Geometry check sheet. Reference: the model listing, model coordinates, mm. A direction names the side the tool comes from. Round coordinates to 2 decimals unless told otherwise and drop trailing zeros. Return JSON: item names as keys, results as strings.
```python
from build123d import *
from build123d.topology import SkipClean

# Parameters (mm, degrees)
SKETCH1_R                    = 27.5
BOSS_EXTRUDE1_DEPTH          = 2
SKETCH2_R                    = 25
BOSS_EXTRUDE2_DEPTH          = 6.5
SKETCH3_R                    = 13
CUT_EXTRUDE1_DEPTH           = 5
SKETCH4_R                    = 11.5
CUT_EXTRUDE2_DEPTH           = 8.5
CHAMFER1_SIZE                = 1
SKETCH5_R                    = 1.55
CUT_EXTRUDE3_DEPTH           = 8.5
SKETCH6_R                    = 3
CUT_EXTRUDE4_DEPTH           = 6
CHAMFER2_SIZE                = 1
CIRPATTERN1_COUNT            = 6
CHAMFER2_OF_CIRPATTERN1_SIZE = 1
SKETCH7_R                    = 1.55
CUT_EXTRUDE5_DEPTH           = 8.5
SKETCH8_R                    = 2.15
CUT_EXTRUDE6_DEPTH           = 4.5
CIRPATTERN2_COUNT            = 6
SKETCH9_R                    = 2.5
SKETCH9_R_2                  = 1.55
BOSS_EXTRUDE3_DEPTH          = 2
CIRPATTERN3_COUNT            = 6


with BuildPart() as part:
    # Sketch1 → Boss-Extrude1 (new body)
    with BuildSketch(Plane(origin=(0, 0, 0), x_dir=(1, 0, 0), z_dir=(0, 1, 0))):
        with Locations(Location((0, 0, 0), (0, 0, 270))):
            Circle(SKETCH1_R)
    extrude(amount=BOSS_EXTRUDE1_DEPTH)

    # Sketch2 → Boss-Extrude2 (add)
    with BuildSketch(Plane(origin=(0, 2, 0), x_dir=(1, 0, 0), z_dir=(0, 1, 0))):
        with Locations(Location((0, 0, 0), (0, 0, 90))):
            Circle(SKETCH2_R)
    extrude(amount=BOSS_EXTRUDE2_DEPTH)

    # Sketch3 → Cut-Extrude1 (cut)
    with BuildSketch(Plane(origin=(0, 8.5, 0), x_dir=(1, 0, 0), z_dir=(0, 1, 0))):
        with Locations(Location((0, 0, 0), (0, 0, 270))):
            Circle(SKETCH3_R)
    extrude(amount=-CUT_EXTRUDE1_DEPTH, mode=Mode.SUBTRACT)

    # Sketch4 → Cut-Extrude2 (cut)
    with BuildSketch(Plane(origin=(0, 8.5, 0), x_dir=(1, 0, 0), z_dir=(0, 1, 0))):
        with Locations(Location((0, 0, 0), (0, 0, 270))):
            Circle(SKETCH4_R)
    extrude(amount=-CUT_EXTRUDE2_DEPTH, mode=Mode.SUBTRACT)

    # Chamfer1
    chamfer1_edges = [part.edges().sort_by_distance(p)[0] for p in [
        (0, 8.5, -13),
        (0, 0, -11.5),
        (0, 0, -27.5),
        (0, 8.5, 25),
    ]]
    chamfer(chamfer1_edges, length=CHAMFER1_SIZE)

    # Sketch5 → Cut-Extrude3 (cut)
    with BuildSketch(Plane.XZ):
        with Locations(Location((0, 21, 0), (0, 0, 270))):
            Circle(SKETCH5_R)
    cut_extrude3 = extrude(amount=-CUT_EXTRUDE3_DEPTH, mode=Mode.SUBTRACT)

    # Sketch6 → Cut-Extrude4 (cut)
    with BuildSketch(Plane.XZ):
        with Locations(Location((0, 21, 0), (0, 0, 270))):
            Circle(SKETCH6_R)
    cut_extrude4 = extrude(amount=-CUT_EXTRUDE4_DEPTH, mode=Mode.SUBTRACT)

    # Chamfer2
    chamfer2_edges = [part.edges().sort_by_distance(p)[0] for p in [
        (0, 0, 24),
    ]]
    chamfer(chamfer2_edges, length=CHAMFER2_SIZE)

    # CirPattern1: Cut-Extrude3, Cut-Extrude4 ×6 about axis
    cirpattern1_axis = Axis((0, 0, 0), (0, 1, 0))
    add([cut_extrude3.rotate(cirpattern1_axis, i * 360 / CIRPATTERN1_COUNT) for i in range(1, CIRPATTERN1_COUNT)], mode=Mode.SUBTRACT)
    add([cut_extrude4.rotate(cirpattern1_axis, i * 360 / CIRPATTERN1_COUNT) for i in range(1, CIRPATTERN1_COUNT)], mode=Mode.SUBTRACT)

    # Chamfer2 of CirPattern1
    chamfer2_of_cirpattern1_edges = [part.edges().sort_by_distance(p)[0] for p in [
        (20.784609691, 0, 12),
        (20.784609691, 0, -12),
        (0, 0, -24),
        (-20.784609691, 0, -12),
        (-20.784609691, 0, 12),
    ]]
    chamfer(chamfer2_of_cirpattern1_edges, length=CHAMFER2_OF_CIRPATTERN1_SIZE)

    # Sketch7 → Cut-Extrude5 (cut)
    with BuildSketch(Plane(origin=(0, 8.5, 0), x_dir=(1, 0, 0), z_dir=(0, 1, 0))):
        with Locations(Location((-10.5, 18.186533479, 0), (0, 0, 270))):
            Circle(SKETCH7_R)
    cut_extrude5 = extrude(amount=-CUT_EXTRUDE5_DEPTH, mode=Mode.SUBTRACT)

    # Sketch8 → Cut-Extrude6 (cut)
    with BuildSketch(Plane(origin=(0, 8.5, 0), x_dir=(1, 0, 0), z_dir=(0, 1, 0))):
        with Locations(Location((-10.5, 18.186533479, 0), (0, 0, 270))):
            Circle(SKETCH8_R)
    cut_extrude6 = extrude(amount=-CUT_EXTRUDE6_DEPTH, mode=Mode.SUBTRACT)

    # CirPattern2: Cut-Extrude5, Cut-Extrude6 ×6 about axis
    cirpattern2_axis = Axis((0, 0, 0), (0, 1, 0))
    add([cut_extrude5.rotate(cirpattern2_axis, i * 360 / CIRPATTERN2_COUNT) for i in range(1, CIRPATTERN2_COUNT)], mode=Mode.SUBTRACT)
    add([cut_extrude6.rotate(cirpattern2_axis, i * 360 / CIRPATTERN2_COUNT) for i in range(1, CIRPATTERN2_COUNT)], mode=Mode.SUBTRACT)

    # Sketch9 → Boss-Extrude3 (add)
    with SkipClean():  # the faces are left unmerged after this step: merging them gives an invalid solid
        with BuildSketch(Plane(origin=(0, 8.5, 0), x_dir=(1, 0, 0), z_dir=(0, 1, 0))):
            with Locations(Location((0, 21, 0), (0, 0, 270))):
                Circle(SKETCH9_R)
            with Locations(Location((0, 21, 0), (0, 0, 90))):
                Circle(SKETCH9_R_2, mode=Mode.SUBTRACT)
        boss_extrude3 = extrude(amount=BOSS_EXTRUDE3_DEPTH)
    add(part.part.scale(1), mode=Mode.REPLACE)  # the faces are merged on a copy

    # CirPattern3: Boss-Extrude3 ×6 about axis
    cirpattern3_axis = Axis((0, 0, 0), (0, 1, 0))
    for i in range(1, CIRPATTERN3_COUNT):
        add(boss_extrude3.rotate(cirpattern3_axis, i * 360 / CIRPATTERN3_COUNT))


solid = part.part
```
(1) Material ranges on line 1 along X through (y, z) = (1.7, 0); line 2 along Z through (x, y) = (3, 6.5); line 3 along X through (y, z) = (1, 13), recorded low to high. Write a range as [from, to].
Response values:
{"line 1": "x = [-27.5, -22.55], [-19.45, -11.5], [11.5, 19.45], [22.55, 27.5]", "line 2": "z = [-24.82, -12.65], [12.65, 24.82]", "line 3": "x = [-24.23, -19.84], [-16.53, 16.53], [19.84, 24.23]"}
(2) Access from +Z, -Z, +X, -X, +Y, -Y to the whole of each face (thin tool, end or side, straight path). Record for faces 1 (the face through (17.7, 6, -8.7)), 2 (the face through (16.665, 9.486, 8.516)), 3 (the face through (-5.5, 0, 11.4)).
Response values:
{"face 1": "-Y", "face 2": "+Y", "face 3": "+Z, -Z, +X, -X, -Y"}
(3) Gauge pin test, flat ends, axial feed: pin 1 (4 mm diameter, centred on y = 3.5, z = -6.5, fed in from -X); pin 2 (1 mm diameter, centred on y = 1, z = 11.5, fed in from +X); pin 3 (6 mm diameter, centred on x = -7.5, y = 2.5, fed in from +Z); pin 4 (2.5 mm diameter, centred on x = 0, z = 21, fed in from +Y). Record the tip position at first contact, or that the pin passes through.
Response values:
{"pin 1": "stops at x = -27.01", "pin 2": "stops at x = 25.2", "pin 3": "stops at z = 27.12", "pin 4": "passes through"}
(4) Release check for a two-part mould opening along X. For faces 4 (the face through (10.3, 8.5, -10.3)), 5 (the face through (-18.9, 6.28, 0.47)), 6 (the face through (-2, 10.5, -21)), 7 (the face through (-7.509, 4.712, -23.846)) record: pulls with the +X half, pulls with the -X half, needs draft (parallel to the pull), parting line crosses it, or undercut.
Response values:
{"face 4": "undercut", "face 5": "undercut", "face 6": "needs draft", "face 7": "parting line crosses it"}
(5) Section check A-A, the plane y = 9.25. Give the number of separate pieces and of enclosed holes in the cut face, plus the area to 3 significant figures.
Response values:
{"separate pieces": "6", "enclosed holes": "6", "area": "72.5 mm^2"}
